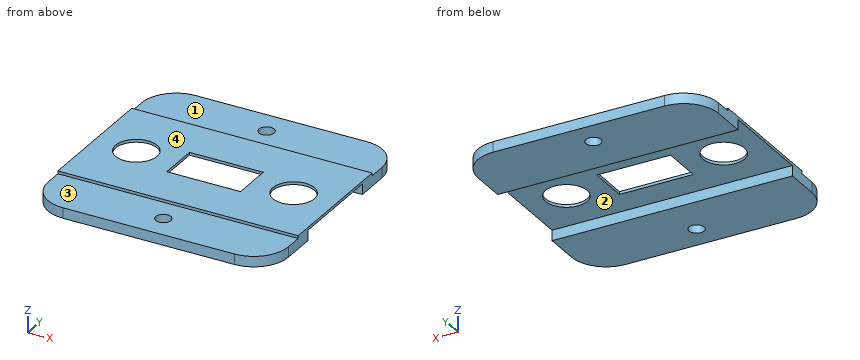
```python
from build123d import *

# Parameters (mm, degrees)
BOSS_EXTRUDE1_DEPTH   = 1.905
BOSS_EXTRUDE1_2_DEPTH = 1.905
SKETCH2_W             = 44.1071
SKETCH2_H             = 24.0792
SKETCH2_R             = 3.81
BOSS_EXTRUDE2_DEPTH   = 0.508
F_3_CLEARANCE_HOLE1_D = 2.794


with BuildPart() as part:
    # Sketch1 → Boss-Extrude1 (new body)
    with BuildSketch(Plane.XY):
        with BuildLine():
            Line((-26.756249968, -18.6229), (-26.756249968, -12.2729))
            ThreePointArc((-26.756249968, -12.2729), (-24.896378028, -7.782771939), (-20.406249968, -5.9229))
            Line((-20.406249968, -5.9229), (11.000850032, -5.9229))
            ThreePointArc((11.000850032, -5.9229), (15.490978093, -7.782771939), (17.350850032, -12.2729))
            Line((17.350850032, -12.2729), (17.350850032, -18.6229))
            Line((17.350850032, -18.6229), (-26.756249968, -18.6229))
        make_face()
    extrude(amount=BOSS_EXTRUDE1_DEPTH)



with BuildPart() as body_2:
    # Sketch1 → Boss-Extrude1 2 (new body)
    with BuildSketch(Plane.XY):
        with BuildLine():
            Line((-26.756249968, -36.3521), (17.350850032, -36.3521))
            Line((17.350850032, -36.3521), (17.350850032, -42.7021))
            ThreePointArc((17.350850032, -42.7021), (15.490978093, -47.192228061), (11.000850032, -49.0521))
            Line((11.000850032, -49.0521), (-20.406249968, -49.0521))
            ThreePointArc((-20.406249968, -49.0521), (-24.896378028, -47.192228061), (-26.756249968, -42.7021))
            Line((-26.756249968, -42.7021), (-26.756249968, -36.3521))
        make_face()
    extrude(amount=BOSS_EXTRUDE1_2_DEPTH)


with BuildPart() as part_1:
    add(part.part)

    add(body_2.part)  # Boss-Extrude2 merges body 2
    # Sketch2 → Boss-Extrude2 (add)
    with BuildSketch(Plane.XY.offset(1.905)):
        with Locations((-4.702699968, -27.4875)):
            Rectangle(SKETCH2_W, SKETCH2_H)
        with Locations((9.730850032, -27.4875)):
            Circle(SKETCH2_R, mode=Mode.SUBTRACT)
        with Locations((-19.136249968, -27.4875)):
            Circle(SKETCH2_R, mode=Mode.SUBTRACT)
        Polygon((-11.478149968, -23.77275), (-11.478149968, -24.71255), (-11.478149968, -30.26245), (-11.478149968, -31.20225), (2.072750032, -31.20225), (2.072750032, -23.77275), align=None, mode=Mode.SUBTRACT)
    extrude(amount=BOSS_EXTRUDE2_DEPTH)

    # #3 Clearance Hole1 (through all)
    with Locations(Plane.XY.offset(1.905)):
        with Locations((-4.702699968, -10.6854), (-4.702699968, -44.2896)):
            Hole(F_3_CLEARANCE_HOLE1_D / 2)


solid = part_1.part
```
Read the model definition and answer for the solid it produces. Units are mm, in the model's axes. Face numbers are marked on the shaded views. A direction names the side the tool comes from. Coordinates: 2 decimals unless noted, no trailing zeros. Loops run counter-clockwise (first coordinate to the right, second up) from the corner with the lowest first, then second, coordinate; pieces in that order, holes last. Notation, with made-up numbers: (10, 73.25) - (27, 73.25) arc R27 cw to (27, 112.25) - close; hole circle Ø3 at (80.5, -36.5). An arc over 180 degrees is marked (long way). Answer in a Markdown table with one row per item.
1. Straight lines are drawn through the part: line 1 (Y direction, x = -16.5, z = 1.25); line 2 (Y direction, x = -6, z = 1.95); line 3 (X direction, y = -29.5, z = 2.1). For each, find the intervals that lie inside material, in ascending order.
Conclusion:
| item | result |
|---|---|
| line 1 | y = -49.05 to -36.35, -18.62 to -5.92 |
| line 2 | y = -39.53 to -31.2, -23.77 to -15.45 |
| line 3 | x = -26.76 to -22.37, -15.9 to -11.48, 2.07 to 6.5, 12.97 to 17.35 |
2. Given pin 1 (3.5 mm diameter, centred on x = -4.7, y = -10.69, fed in from +Z) (3 decimals); pin 2 (2 mm diameter, centred on x = -5.5, y = -24.5, fed in from -Z) (3 decimals), each flat-ended and moving along its own axis, determine where each tip first touches the part or whether it passes through.
Conclusion:
| item | result |
|---|---|
| pin 1 | stops at z = 1.905 |
| pin 2 | stops at z = 1.905 |
3. Find section B-B, the plane z = 1.1. Write down the section's boundary in (x, y).
Conclusion:
| item | result |
|---|---|
| outline | (-26.76, -42.7) arc R6.35 ccw to (-20.41, -49.05) - (11, -49.05) arc R6.35 ccw to (17.35, -42.7) - (17.35, -36.35) - (-26.76, -36.35) - close; (-26.76, -18.62) - (17.35, -18.62) - (17.35, -12.27) arc R6.35 ccw to (11, -5.92) - (-20.41, -5.92) arc R6.35 ccw to (-26.76, -12.27) - close; hole circle Ø2.79 at (-4.7, -44.29); hole circle Ø2.79 at (-4.7, -10.69) |
4. Which of the six approach directions +Z, -Z, +X, -X, +Y, -Y give full straight-line access (tool end or side, diameter ignored) to the marked faces 3 and 4?
Conclusion:
| item | result |
|---|---|
| face 3 | +Z, +X, -X, -Y |
| face 4 | +Z, +X, -X, +Y, -Y |
5. Find section C-C, the plane y = -26. Write down the section's boundary in (x, z) (3 decimals).
Conclusion:
| item | result |
|---|---|
| outline | (-26.756, 1.905) - (-22.644, 1.905) - (-22.644, 2.413) - (-26.756, 2.413) - close; (-15.629, 1.905) - (-11.478, 1.905) - (-11.478, 2.413) - (-15.629, 2.413) - close; (2.073, 1.905) - (6.223, 1.905) - (6.223, 2.413) - (2.073, 2.413) - close; (13.238, 1.905) - (17.351, 1.905) - (17.351, 2.413) - (13.238, 2.413) - close |
6. Find section A-A, the plane x = -8. Write down the section's boundary in (y, z) (3 decimals), then the cut area to 3 significant figures.
Conclusion:
| item | result |
|---|---|
| outline | (-49.052, 0) - (-36.352, 0) - (-36.352, 1.905) - (-31.202, 1.905) - (-31.202, 2.413) - (-39.527, 2.413) - (-39.527, 1.905) - (-49.052, 1.905) - close; (-23.773, 1.905) - (-18.623, 1.905) - (-18.623, 0) - (-5.923, 0) - (-5.923, 1.905) - (-15.448, 1.905) - (-15.448, 2.413) - (-23.773, 2.413) - close |
| area | 56.8 mm² |
7. Determine the mould class of the marked faces 1 and 2 for opening direction Y: +Y half, -Y half, draft (parallel to the pull), parting line (faces both ways), or undercut.
Conclusion:
| item | result |
|---|---|
| face 1 | draft |
| face 2 | undercut |
8. Find section D-D, the plane x = -14. Write down the section's boundary in (y, z) (3 decimals).
Conclusion:
| item | result |
|---|---|
| outline | (-49.052, 0) - (-36.352, 0) - (-36.352, 1.905) - (-18.623, 1.905) - (-18.623, 0) - (-5.923, 0) - (-5.923, 1.905) - (-15.448, 1.905) - (-15.448, 2.413) - (-39.527, 2.413) - (-39.527, 1.905) - (-49.052, 1.905) - close |
